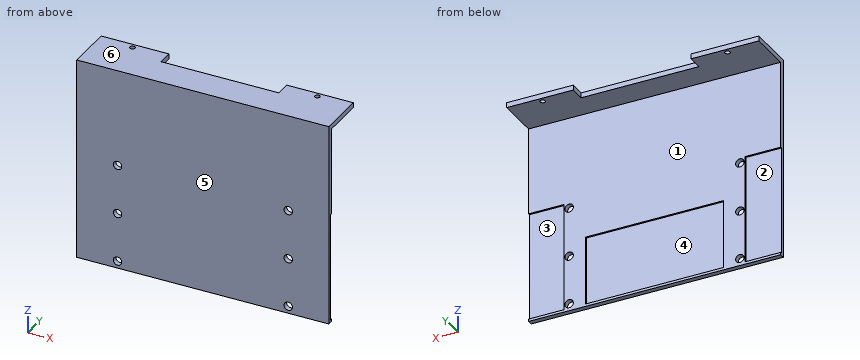
from build123d import *

# Parameters (mm, degrees)
BOSS_EXTRUDE1_DEPTH = 150
SKETCH2_W           = 70
SKETCH2_H           = 9.077653183
CUT_EXTRUDE2_DEPTH  = 3
SKETCH3_W           = 21.1
SKETCH3_H           = 64.5
CUT_EXTRUDE3_DEPTH  = 1
SKETCH4_W           = 82
SKETCH4_H           = 41
CUT_EXTRUDE4_DEPTH  = 1
SKETCH5_R           = 2.5
CUT_EXTRUDE5_DEPTH  = 3
SKETCH6_R           = 1.5
CUT_EXTRUDE6_DEPTH  = 3


with BuildPart() as part:
    # Sketch1 → Boss-Extrude1 (new body)
    with BuildSketch(Plane(origin=(0, 0, 0), x_dir=(0, 0, -1), z_dir=(1, 0, 0))):
        Polygon((-70.218878969, 2.934000234), (-70.218878969, 30.934000234), (-67.218878969, 30.934000234), (-67.218878969, 5.934000234), (50.781121031, 5.934000234), (50.781121031, 2.934000234), align=None)
    extrude(amount=-BOSS_EXTRUDE1_DEPTH)

    # Sketch2 → Cut-Extrude2 (cut)
    with BuildSketch(Plane.XY.offset(70.218878969)):
        with Locations((-74.626034168, 26.395173643)):
            Rectangle(SKETCH2_W, SKETCH2_H)
    extrude(amount=-CUT_EXTRUDE2_DEPTH, mode=Mode.SUBTRACT)

    # Sketch3 → Cut-Extrude3 (cut)
    with BuildSketch(Plane(origin=(0, 5.934000234, 0), x_dir=(1, 0, 0), z_dir=(0, 1, 0))):
        with Locations((-10.55, 17.081121031)):
            Rectangle(SKETCH3_W, SKETCH3_H)
        with Locations((-139.45, 17.081121031)):
            Rectangle(SKETCH3_W, SKETCH3_H)
    extrude(amount=-CUT_EXTRUDE3_DEPTH, mode=Mode.SUBTRACT)

    # Sketch4 → Cut-Extrude4 (cut)
    with BuildSketch(Plane(origin=(0, 5.934000234, 0), x_dir=(1, 0, 0), z_dir=(0, 1, 0))):
        with Locations((-75, 28.831121031)):
            Rectangle(SKETCH4_W, SKETCH4_H)
    extrude(amount=-CUT_EXTRUDE4_DEPTH, mode=Mode.SUBTRACT)

    # Sketch5 → Cut-Extrude5 (cut)
    with BuildSketch(Plane(origin=(0, 5.934000234, 0), x_dir=(1, 0, 0), z_dir=(0, 1, 0))):
        with Locations(Location((-24.143437735, -12.14833258, 0), (0, 0, 270))):
            Circle(SKETCH5_R)
        with Locations(Location((-24.143437735, 46.482481241, 0), (0, 0, 270))):
            Circle(SKETCH5_R)
        with Locations(Location((-24.143437735, 17.329037904, 0), (0, 0, 270))):
            Circle(SKETCH5_R)
        with Locations(Location((-125.69459869, 46.482481241, 0), (0, 0, 270))):
            Circle(SKETCH5_R)
        with Locations(Location((-125.69459869, 17.329037904, 0), (0, 0, 270))):
            Circle(SKETCH5_R)
        with Locations(Location((-125.69459869, -12.14833258, 0), (0, 0, 270))):
            Circle(SKETCH5_R)
    extrude(amount=-CUT_EXTRUDE5_DEPTH, mode=Mode.SUBTRACT)

    # Sketch6 → Cut-Extrude6 (cut)
    with BuildSketch(Plane.XY.offset(70.218878969)):
        with Locations((-129.813017084, 27.934000234)):
            Circle(SKETCH6_R)
        with Locations((-19.813017084, 27.934000234)):
            Circle(SKETCH6_R)
    extrude(amount=-CUT_EXTRUDE6_DEPTH, mode=Mode.SUBTRACT)


solid = part.part
The listing builds one solid part. Answer for the finished solid, in the listing's coordinates (mm). Face numbers are marked on the shaded views. A direction names the side the tool comes from. Round coordinates to 2 decimals unless told otherwise and drop trailing zeros. Loops run counter-clockwise (first coordinate to the right, second up) from the corner with the lowest first, then second, coordinate; pieces in that order, holes last. Notation, with made-up numbers: M -5,-31.75 L 31,-31.75 A21 cw 31,-16.75 Z; hole C 34,42 d4. An arc over 180 degrees is marked long. Write each question's results on one line, items separated by ' | '. Start each with the question number.
1) Straight lines are drawn through the part: probe 1 along Y at (x, z) = (-129, 15.5); probe 2 along Z at (x, y) = (-12, 29.5); probe 3 along Y at (x, z) = (-134, -26). For each, find the intervals that lie inside material, in ascending order.
2) Each of these flat-tipped pins is pushed along its axis until it touches: pin 1 (12.5 mm diameter, centred on x = -75.5, z = -28, fed in from +Y); pin 2 (8 mm diameter, centred on x = -125.69, z = 12.15, fed in from +Y); pin 3 (5 mm diameter, centred on x = -133, y = 12, fed in from -Z). Where does it stop, or does it pass through?
3) Find section B-B on x = -119. Write down the section's boundary in (y, z), plus the area to 3 significant figures.
4) Find section C-C on z = 12.5. Write down the section's boundary in (x, y).
5) Find section A-A on y = 23.5. Write down the section's boundary in (x, z).
6) Find section D-D on z = 36.5. Write down the section's boundary in (x, y), plus the area to 3 significant figures.
7) Which of the six approach directions +Z, -Z, +X, -X, +Y, -Y give full straight-line access (tool end or side, diameter ignored) to the marked faces 1 and 2?
8) Determine the mould class of the marked faces 3, 4, 5 and 6 for opening direction Z: pulls with the +Z half, pulls with the -Z half, needs draft (parallel to the pull), parting line crosses it, or undercut.
Final values:
1) probe 1: 2.93 to 5.93 | probe 2: 67.22 to 70.22 | probe 3: 2.93 to 4.93
2) pin 1: y = 4.93 | pin 2: y = 5.93 | pin 3: z = 67.22
3) outline: M 2.93,-50.78 L 5.93,-50.78 L 5.93,67.22 L 30.93,67.22 L 30.93,70.22 L 2.93,70.22 Z | area: 438 mm²
4) outline: M -150,2.93 L -128.17,2.93 L -128.17,5.93 L -128.9,5.93 L -128.9,4.93 L -150,4.93 Z; M -123.22,2.93 L -26.62,2.93 L -26.62,5.93 L -123.22,5.93 Z; M -21.67,2.93 L 0,2.93 L 0,4.93 L -21.1,4.93 L -21.1,5.93 L -21.67,5.93 Z
5) outline: M -150,67.22 L -109.63,67.22 L -109.63,70.22 L -150,70.22 Z; M -39.63,67.22 L 0,67.22 L 0,70.22 L -39.63,70.22 Z
6) outline: M -150,2.93 L 0,2.93 L 0,5.93 L -150,5.93 Z | area: 450 mm²
7) face 1: -Z, +X, -X, +Y | face 2: -X, +Y
8) face 3: undercut | face 4: undercut | face 5: needs draft | face 6: pulls with the +Z half
